The listing builds one solid part. Answer for the finished solid, in the listing's coordinates (mm). Face numbers are marked on the shaded views. Give positions to 0.01 mm unless a question says otherwise; leave off trailing zeros. Loops run counter-clockwise (first coordinate to the right, second up) from the corner with the lowest first, then second, coordinate; pieces in that order, holes last.
Item 1: Consider line 1 along X through (y, z) = (-2.5, 0); line 2 along Z through (x, y) = (0, -2.45); line 3 along X through (y, z) = (0.6, 0.5). Determine where each line is inside the solid, lowest interval first.
Item 2: Section B-B, the plane x = -2 is taken. Give the vertices of the cut face in (y, z).
Item 3: Section A-A, the plane x = 3.25 is taken. Give the vertices of the cut face in (y, z), and give its area (3 significant figures).
Item 4: The mould has two halves that part along Z. Classify the marked faces 1, 2 and 3: pulls with the +Z half, pulls with the -Z half, needs draft (parallel to the pull), parting line crosses it, or undercut.
Item 5: Each of these flat-tipped pins is pushed along its axis until it touches: pin 1 Ø2 at (x, y) = (3, 1.5) entering from +Z; pin 2 Ø1 at (x, z) = (-0.5, 0) entering from -Y. Where does it stop, or does it pass through?
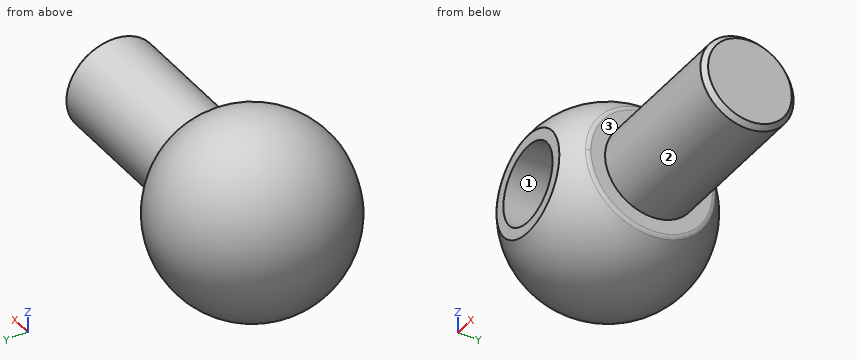
from build123d import *

# Parameters (mm, degrees)
SKETCH_2_R             = 2
CUT_EXTRUDE_1_DEPTH    = 7.77
SKETCH_3_R             = 1.48
EXTRUDE_1_DEPTH        = 5
FILLET_2_R             = 0.2
FILLET_3_R             = 0.2
CHAMFER_1_SIZE         = 0.15
SKETCH_4_R             = 1.6
CUT_EXTRUDE_3_DEPTH    = 2.465
HOLE_WIZARD_M3_2_D     = 2.5
HOLE_WIZARD_M3_2_DEPTH = 4
HOLE_WIZARD_M3_2_TIP   = 0.7510757737844503


# Some blends are built 0.0001 mm under size
with BuildPart() as part:
    # 草图1 → 旋转1 (revolve)
    with BuildSketch(Plane.XY):
        with BuildLine():
            Line((0, 2.999999999999999), (0, -2.999999999999999))
            ThreePointArc((0, -2.999999999999999), (2.999999999999999, 0), (0, 2.999999999999999))
        make_face()
    revolve(axis=Axis((0, 2.999999999999999, 0), (0, -1, 0)))

    # 草图2 → 切除-拉伸1 (cut)
    with BuildSketch(Plane(origin=(10, 0, 0), x_dir=(0, 0, -1), z_dir=(1, 0, 0))):
        Circle(SKETCH_2_R)
    extrude(amount=-CUT_EXTRUDE_1_DEPTH, mode=Mode.SUBTRACT)

    # 草图3 → 凸台-拉伸1 (add)
    with BuildSketch(Plane(origin=(2.2300000000000004, 0, 0), x_dir=(0, 0, -1), z_dir=(1, 0, 0))):
        Circle(SKETCH_3_R)
    extrude(amount=EXTRUDE_1_DEPTH)

    # 圆角2
    # the kernel refuses this fillet: 0.2 mm, written as the material it takes off along each edge
    with BuildSketch(Plane(origin=(2.236067977499788, 0, 0), x_dir=(0, 1, -1.8e-16), z_dir=(0, -1.8e-16, -1))) as fillet_2_piece_1:
        with BuildLine():
            CenterArc((1.8997145722011748, -0.17910795256821466), FILLET_2_R, 47.27584094143335, 12.629695301093555)
            Line((1.9999999999994043, -0.00606797750081567), (2, 0))
            ThreePointArc((2, 0), (2.0177683971304545, -0.0160205240561484), (2.0354084702155446, -0.03218223650167351))
        make_face()
    revolve(axis=Axis((2.236067977499788, 0, 0), (1, 0, 0)), revolution_arc=180, mode=Mode.SUBTRACT)
    with BuildSketch(Plane(origin=(2.236067977499788, 0, 0), x_dir=(0, -5.7e-16, -1), z_dir=(0, -1, 5.7e-16))) as fillet_2_piece_2:
        with BuildLine():
            CenterArc((1.8997145722011737, -0.17910795256821377), FILLET_2_R, 47.2758409414334, 12.629695301093115)
            Line((1.9999999999994045, -0.00606797750081522), (2, 0))
            ThreePointArc((2, 0), (2.0177683971304545, -0.01602052405614884), (2.0354084702155433, -0.03218223650167262))
        make_face()
    revolve(axis=Axis((2.236067977499788, 0, 0), (1, 0, 0)), revolution_arc=90.00000000000003, mode=Mode.SUBTRACT)
    with BuildSketch(Plane(origin=(2.236067977499788, 0, 0), x_dir=(0, -1, 6e-17), z_dir=(0, 6e-17, 1))) as fillet_2_piece_3:
        with BuildLine():
            CenterArc((1.8997145722011748, -0.17910795256821466), FILLET_2_R, 47.27584094143335, 12.629695301093555)
            Line((1.9999999999994043, -0.00606797750081567), (2, 0))
            ThreePointArc((2, 0), (2.0177683971304545, -0.0160205240561484), (2.0354084702155446, -0.03218223650167351))
        make_face()
    revolve(axis=Axis((2.236067977499788, 0, 0), (1, 0, 0)), revolution_arc=89.99999999999997, mode=Mode.SUBTRACT)

    # 圆角3
    fillet_3_edges = [part.edges().sort_by_distance(p)[0] for p in [
        (2.2299999999999995, -8.1e-16, 1.9999999999999996),
    ]]
    fillet(fillet_3_edges, radius=FILLET_3_R - 0.0001)  # a hair under: the kernel refuses the full size

    # 倒角1
    chamfer_1_edges = [part.edges().sort_by_distance(p)[0] for p in [
        (7.23, -4.8e-16, 1.48),
    ]]
    chamfer(chamfer_1_edges, length=CHAMFER_1_SIZE)

    # 草图4 → 切除-拉伸3 (cut)
    with BuildSketch(Plane(origin=(0, -5, 0), x_dir=(-1, 0, 0), z_dir=(0, 1, 0))):
        with Locations(Location((0, 0, 0), (0, 0, 90))):
            Circle(SKETCH_4_R)
    extrude(amount=CUT_EXTRUDE_3_DEPTH, mode=Mode.SUBTRACT)

    # M3 螺纹孔2
    with Locations(Plane(origin=(0, -2.535, 0), x_dir=(0, 0, -1), z_dir=(0, -1, 0))):
        with Locations((0, 0)):
            Hole(HOLE_WIZARD_M3_2_D / 2, depth=HOLE_WIZARD_M3_2_DEPTH)
            with Locations((0, 0, -(HOLE_WIZARD_M3_2_DEPTH + HOLE_WIZARD_M3_2_TIP / 2))):  # 118° drill point
                Cone(0, HOLE_WIZARD_M3_2_D / 2, HOLE_WIZARD_M3_2_TIP, mode=Mode.SUBTRACT)


solid = part.part
Worked answers:
1. line 1: x = -1.66 to -1.25, 1.25 to 1.66
1. line 2: z = -1.73 to -1.25, 1.25 to 1.73
1. line 3: x = -2.9 to -1.15, 1.15 to 7.23
2. outline: circle Ø4.47 at (0, 0)
3. outline: circle Ø2.96 at (0, 0)
3. area: 6.88 mm2
4. face 1: undercut
4. face 2: parting line crosses it
4. face 3: needs draft
5. pin 1: stops at z = 1.86
5. pin 2: stops at y = 1.62
